```python
from build123d import *

# Parameters (mm, degrees)
BOSS_EXTRUDE1_DEPTH   = 44
BOSS_EXTRUDE2_DEPTH   = 15
BOSS_EXTRUDE3_DEPTH   = 22
BOSS_EXTRUDE4_START   = 10
BOSS_EXTRUDE4_DEPTH   = 24
FILLET3_RADIUS        = 12
FILLET3_LENGTH        = 9
FILLET4_RADIUS        = 12
FILLET4_LENGTH        = 9
F_6_0MM_DOWEL_HOLE1_D = 6


with BuildPart() as part:
    # Sketch1 → Boss-Extrude1 (new body)
    with BuildSketch(Plane.XY):
        with BuildLine():
            Line((0, 25.5), (-2.000483947, 25.421409559))
            ThreePointArc((-2.000483947, 25.421409559), (-25.5, 0), (-2.000483947, -25.421409559))
            Line((-2.000483947, -25.421409559), (0, -25.5))
            ThreePointArc((0, -25.5), (14.05791592, -21.274985311), (23.457408211, -10))
            ThreePointArc((23.457408211, -10), (24.879246203, -5.592236438), (25.480384612, -1))
            Line((25.480384612, -1), (15.838462678, -1))
            ThreePointArc((15.838462678, -1), (-15.87, 0), (15.838462678, 1))
            Line((15.838462678, 1), (25.480384612, 1))
            ThreePointArc((25.480384612, 1), (24.879246203, 5.592236438), (23.457408211, 10))
            ThreePointArc((23.457408211, 10), (14.05791592, 21.274985311), (0, 25.5))
        make_face()
    extrude(amount=BOSS_EXTRUDE1_DEPTH)

    # Sketch1<3> → Boss-Extrude2 (add)
    with BuildSketch(Plane.XY):
        with BuildLine():
            Line((-2.000483947, 25.421409559), (-140, 20))
            Line((-140, 20), (-90, 20))
            ThreePointArc((-90, 20), (-70, 0), (-90, -20))
            Line((-90, -20), (-140, -20))
            Line((-140, -20), (-2.000483947, -25.421409559))
            ThreePointArc((-2.000483947, -25.421409559), (-25.5, 0), (-2.000483947, 25.421409559))
        make_face()
    extrude(amount=BOSS_EXTRUDE2_DEPTH)

    # Sketch1<4> → Boss-Extrude3 (add)
    with BuildSketch(Plane.XY):
        with BuildLine():
            Line((-140, -20), (-90, -20))
            ThreePointArc((-90, -20), (-70, 0), (-90, 20))
            Line((-90, 20), (-140, 20))
            ThreePointArc((-140, 20), (-160, 0), (-140, -20))
        make_face()
        with BuildLine():
            ThreePointArc((-90, -6), (-84, 0), (-90, 6))
            Line((-90, 6), (-140, 6))
            ThreePointArc((-140, 6), (-146, 0), (-140, -6))
            Line((-140, -6), (-90, -6))
        make_face(mode=Mode.SUBTRACT)
    extrude(amount=BOSS_EXTRUDE3_DEPTH)

    # Sketch1<5> → Boss-Extrude4 (add)
    with BuildSketch(Plane.XY.offset(BOSS_EXTRUDE4_START)):
        with BuildLine():
            Line((44, 10), (23.457408211, 10))
            ThreePointArc((23.457408211, 10), (24.879246203, 5.592236438), (25.480384612, 1))
            Line((25.480384612, 1), (44, 1))
            Line((44, 1), (44, 10))
        make_face()
        with BuildLine():
            ThreePointArc((25.480384612, -1), (24.879246203, -5.592236438), (23.457408211, -10))
            Line((23.457408211, -10), (44, -10))
            Line((44, -10), (44, -1))
            Line((44, -1), (25.480384612, -1))
        make_face()
    extrude(amount=BOSS_EXTRUDE4_DEPTH)

    # Fillet3: full round fillet: the end face becomes a half cylinder, R = half its width
    fillet3_face = Plane((44, 5.5, 22), x_dir=(0, 1, 0), z_dir=(1, 0, 0))  # on the end face: x along it, z out of the body
    fillet3_slab = fillet3_face.offset(-FILLET3_RADIUS / 2) * Box(FILLET3_LENGTH, 2 * FILLET3_RADIUS, FILLET3_RADIUS, mode=Mode.PRIVATE)  # the body's end, R deep
    fillet3_round = Plane((32, 5.5, 22), x_dir=(1, 0, 0), z_dir=(0, 1, 0)) * Cylinder(FILLET3_RADIUS, FILLET3_LENGTH, mode=Mode.PRIVATE)  # its axis R under the face
    add(fillet3_slab - fillet3_round, mode=Mode.SUBTRACT)

    # Fillet4: full round fillet: the end face becomes a half cylinder, R = half its width
    fillet4_face = Plane((44, -5.5, 22), x_dir=(0, -1, 0), z_dir=(1, 0, 0))  # on the end face: x along it, z out of the body
    fillet4_slab = fillet4_face.offset(-FILLET4_RADIUS / 2) * Box(FILLET4_LENGTH, 2 * FILLET4_RADIUS, FILLET4_RADIUS, mode=Mode.PRIVATE)  # the body's end, R deep
    fillet4_round = Plane((32, -5.5, 22), x_dir=(1, 0, 0), z_dir=(0, -1, 0)) * Cylinder(FILLET4_RADIUS, FILLET4_LENGTH, mode=Mode.PRIVATE)  # its axis R under the face
    add(fillet4_slab - fillet4_round, mode=Mode.SUBTRACT)

    # Ø6.0mm Dowel Hole1 (through all)
    with Locations(Plane(origin=(34.387865252, 10, 21.746882561), x_dir=(1, 0, 0), z_dir=(0, 1, 0))):
        with Locations((0, 0)):
            Hole(F_6_0MM_DOWEL_HOLE1_D / 2)


solid = part.part
```
Here's how the part is built. I have some questions about the finished solid (model axes, mm). A direction names the side the tool comes from. Round coordinates to 2 decimals unless told otherwise and drop trailing zeros. Order: outer loops, then holes, each group sorted by start corner. A loop starts at its lowest first (then second) coordinate and runs counter-clockwise, first axis right, second up. Notation, with made-up numbers: (26, 57) -> (68, 57) arc R20 cw to (68, 65) -> close; hole circle Ø3 at (-13, 72). An arc over 180 degrees is marked (long way). Use a Markdown table: item, result. Add a question column.
(1) For pin 1 Ø3 at (y, z) = (-1, 10.5) entering from +X; pin 2 Ø24 at (x, z) = (-115.5, 14.5) entering from -Y; pin 3 Ø10 at (y, z) = (20, 34.5) entering from +X, each with a flat end and sliding along its axis, tell me the tip position at first contact or that it passes through.
(2) For faces 1 (the face through (-115, 20, 18)), 2 (the face through (32, 10, 24)), 3 (the face through (-84, 0, 11)), 4 (the face through (-116, 9, 22)), 5 (the face through (-69, 0, 0)), which set-ups out of +Z, -Z, +X, -X, +Y, -Y let a thin tool reach every point of the face, with its end or its side?
(3) If we mould it in two halves opening along X, with no side actions, what happens to faces 6 (the face through (-70, 0, 18)), 7 (the face through (-25.494, 0.533, 29.297)), 8 (the face through (31, -10, 22)), 9 (the face through (44, -6, 22))? For each: released by +X, released by -X, zero draft, split by the parting line, or undercut.
(4) Suppose I cut it at D-D, the plane z = 30. Please give me the cut outline in (x, y).
(5) I need wall thicknesses on line 1 along Y through (x, z) = (-140, 5); line 2 along Y through (x, z) = (0, 29); line 3 along Z through (x, y) = (-10, 23.5). Which ranges of each line are inside material? Lowest first, please.
(6) Suppose I cut it at A-A, the plane z = 3. Please give me the cut outline in (x, y), and give its area (3 significant figures).
(7) Suppose I cut it at C-C, the plane y = 3.5. Please give me the cut outline in (x, z).
(8) Suppose I cut it at B-B, the plane y = -8. Please give me the cut outline in (x, z).
Verdict:
| question | item | result |
|---|---|---|
| 1 | pin 1 | x = 38.63 |
| 1 | pin 2 | y = -21.43 |
| 1 | pin 3 | x = 20.62 |
| 2 | face 1 | +Z, -X, +Y |
| 2 | face 2 | +Z, -Z, +X, +Y |
| 2 | face 3 | +Z, -Z |
| 2 | face 4 | +Z, -X, +Y, -Y |
| 2 | face 5 | -Z, +X, -X, +Y, -Y |
| 3 | face 6 | undercut |
| 3 | face 7 | undercut |
| 3 | face 8 | zero draft |
| 3 | face 9 | released by +X |
| 4 | outline | (-2, -25.42) -> (0, -25.5) arc R25.5 ccw to (23.46, -10) -> (40.94, -10) -> (40.94, -1) -> (15.84, -1) arc R15.87 cw (long way) to (15.84, 1) -> (40.94, 1) -> (40.94, 10) -> (23.46, 10) arc R25.5 ccw to (0, 25.5) -> (-2, 25.42) arc R25.5 ccw to start |
| 5 | line 1 | -20 to -6, 6 to 20 |
| 5 | line 2 | -25.5 to -15.87, 15.87 to 25.5 |
| 5 | line 3 | 0 to 15 |
| 6 | outline | (-140, -20) -> (0, -25.5) arc R25.5 ccw to (25.48, -1) -> (15.84, -1) arc R15.87 cw (long way) to (15.84, 1) -> (25.48, 1) arc R25.5 ccw to (0, 25.5) -> (-140, 20) arc R20 ccw to start; hole (-140, -6) -> (-90, -6) arc R6 ccw to (-90, 6) -> (-140, 6) arc R6 ccw to start |
| 6 | area | 6,500 mm2 |
| 7 | outline | (-159.69, 0) -> (-144.87, 0) -> (-144.87, 22) -> (-159.69, 22) -> close; (-85.13, 0) -> (-15.48, 0) -> (-15.48, 44) -> (-25.26, 44) -> (-25.26, 15) -> (-70.31, 15) -> (-70.31, 22) -> (-85.13, 22) -> close; (15.48, 0) -> (25.26, 0) -> (25.26, 10) -> (32, 10) arc R12 ccw to (32, 34) -> (25.26, 34) -> (25.26, 44) -> (15.48, 44) -> close; hole circle Ø6 at (34.39, 21.75) |
| 8 | outline | (-158.33, 0) -> (-13.71, 0) -> (-13.71, 44) -> (-24.21, 44) -> (-24.21, 15) -> (-71.67, 15) -> (-71.67, 22) -> (-158.33, 22) -> close; (13.71, 0) -> (24.21, 0) -> (24.21, 10) -> (32, 10) arc R12 ccw to (32, 34) -> (24.21, 34) -> (24.21, 44) -> (13.71, 44) -> close; hole circle Ø6 at (34.39, 21.75) |
